from build123d import *

# Parameters (mm, degrees)
SKETCH1_W                   = 33.528
SKETCH1_H                   = 33.02
BOSS_EXTRUDE1_DEPTH         = 3.175
CUT_EXTRUDE1_DEPTH          = 24.742207585
CUT_EXTRUDE2_DEPTH          = 24.742207585
SKETCH4_W                   = 6.08076
SKETCH4_H                   = 5.45338
BOSS_EXTRUDE2_DEPTH         = 6.08076
SKETCH5_W                   = 6.08076
SKETCH5_H                   = 5.45338
BOSS_EXTRUDE3_DEPTH         = 6.08076
SKETCH6_W                   = 6.08076
SKETCH6_H                   = 5.45338
BOSS_EXTRUDE4_DEPTH         = 6.08076
SKETCH7_W                   = 6.08076
SKETCH7_H                   = 5.45338
BOSS_EXTRUDE5_DEPTH         = 6.08076
HOLE1_D                     = 12.7254
M2_5_CLEARANCE_HOLE1_D      = 2.7051
M3_CLEARANCE_HOLE1_D        = 3.556
M2_5_CLEARANCE_HOLE2_D      = 2.7051
M2_5_CLEARANCE_HOLE2_DEPTH  = 39.60876
M2_5_CLEARANCE_HOLE3_D      = 2.7051
M2_5_CLEARANCE_HOLE3_DEPTH  = 39.60876
M2_5_CLEARANCE_HOLE4_REACH  = 27.061
M2_5_CLEARANCE_HOLE4_BORE_R = 1.35255
FILLET1_R                   = 0.635
FILLET2_R                   = 3.04038


with BuildPart() as part:
    # Sketch1 → Boss-Extrude1 (new body)
    with BuildSketch(Plane(origin=(0, 3.175, 0), x_dir=(1, 0, 0), z_dir=(0, 1, 0))):
        Rectangle(SKETCH1_W, SKETCH1_H)
    extrude(amount=-BOSS_EXTRUDE1_DEPTH)

    # Sketch2 → Cut-Extrude1 (cut, through all)
    with BuildSketch(Plane.XZ):
        with BuildLine():
            Line((16.764, -10.42924), (16.764, 10.42924))
            ThreePointArc((16.764, 10.42924), (14.617411383, 9.536940757), (13.7287, 7.388864244))
            Line((13.7287, 7.388864244), (13.7287, -7.388864244))
            ThreePointArc((13.7287, -7.388864244), (14.617411383, -9.536940757), (16.764, -10.42924))
        make_face()
    extrude(amount=-CUT_EXTRUDE1_DEPTH, mode=Mode.SUBTRACT)

    # Sketch3 → Cut-Extrude2 (cut, through all)
    with BuildSketch(Plane.XZ):
        with BuildLine():
            Line((-16.764, 10.42924), (-16.764, -10.42924))
            ThreePointArc((-16.764, -10.42924), (-14.617411383, -9.536940757), (-13.7287, -7.388864244))
            Line((-13.7287, -7.388864244), (-13.7287, 7.388864244))
            ThreePointArc((-13.7287, 7.388864244), (-14.617411383, 9.536940757), (-16.764, 10.42924))
        make_face()
    extrude(amount=-CUT_EXTRUDE2_DEPTH, mode=Mode.SUBTRACT)

    # Sketch4 → Boss-Extrude2 (add)
    with BuildSketch(Plane(origin=(0, 0, -16.51), x_dir=(-1, 0, 0), z_dir=(0, 0, -1))):
        with Locations((13.72362, 5.90169)):
            Rectangle(SKETCH4_W, SKETCH4_H)
    extrude(amount=-BOSS_EXTRUDE2_DEPTH)

    # Sketch5 → Boss-Extrude3 (add)
    with BuildSketch(Plane(origin=(0, 0, -16.51), x_dir=(-1, 0, 0), z_dir=(0, 0, -1))):
        with Locations((-13.72362, 5.90169)):
            Rectangle(SKETCH5_W, SKETCH5_H)
    extrude(amount=-BOSS_EXTRUDE3_DEPTH)

    # Sketch6 → Boss-Extrude4 (add)
    with BuildSketch(Plane.XY.offset(16.51)):
        with Locations((13.72362, 5.90169)):
            Rectangle(SKETCH6_W, SKETCH6_H)
    extrude(amount=-BOSS_EXTRUDE4_DEPTH)

    # Sketch7 → Boss-Extrude5 (add)
    with BuildSketch(Plane.XY.offset(16.51)):
        with Locations((-13.72362, 5.90169)):
            Rectangle(SKETCH7_W, SKETCH7_H)
    extrude(amount=-BOSS_EXTRUDE5_DEPTH)

    # Hole1 (through all)
    with Locations(Plane(origin=(0, 3.175, 0), x_dir=(1, 0, 0), z_dir=(0, 1, 0))):
        with Locations((0, 0)):
            Hole(HOLE1_D / 2)

    # M2.5 Clearance Hole1 (through all)
    with Locations(Plane(origin=(0, 3.175, 0), x_dir=(1, 0, 0), z_dir=(0, 1, 0))):
        with Locations((0, 9.779), (-9.779, 0), (0, -9.779), (9.779, 0)):
            Hole(M2_5_CLEARANCE_HOLE1_D / 2)

    # M3 Clearance Hole1 (through all)
    with Locations(Plane(origin=(0, 3.175, 0), x_dir=(1, 0, 0), z_dir=(0, 1, 0))):
        with Locations((-5.579615818, -13.470384182), (5.579615818, -13.470384182), (5.579615818, 13.470384182), (-5.579615818, 13.470384182), (6.914797213, 6.914797213), (-6.914797213, 6.914797213), (-6.914797213, -6.914797213), (6.914797213, -6.914797213)):
            Hole(M3_CLEARANCE_HOLE1_D / 2)

    # M2.5 Clearance Hole2
    with Locations(Plane(origin=(16.764, 0, 0), x_dir=(0, 0, -1), z_dir=(1, 0, 0))):
        with Locations((-13.470384182, 5.588)):
            Hole(M2_5_CLEARANCE_HOLE2_D / 2, depth=M2_5_CLEARANCE_HOLE2_DEPTH)

    # M2.5 Clearance Hole3
    with Locations(Plane.ZY.offset(16.764)):
        with Locations((-13.470384182, 5.588)):
            Hole(M2_5_CLEARANCE_HOLE3_D / 2, depth=M2_5_CLEARANCE_HOLE3_DEPTH)

    # M2.5 Clearance Hole4 bore → M2.5 Clearance Hole4 (cut, up to next)
    with BuildSketch(Plane(origin=(0, 0, 0), x_dir=(-1, 0, 0), z_dir=(0, -1, 0)), mode=Mode.PRIVATE) as m2_5_clearance_hole4_sk1:
        with Locations((13.470384182, 13.470384182)):
            Circle(M2_5_CLEARANCE_HOLE4_BORE_R)
    m2_5_clearance_hole4_tool1 = extrude(m2_5_clearance_hole4_sk1.sketch, amount=-M2_5_CLEARANCE_HOLE4_REACH, mode=Mode.PRIVATE) & part.part
    # M2.5 Clearance Hole4 bore → M2.5 Clearance Hole4 (cut, up to next)
    with BuildSketch(Plane(origin=(0, 0, 0), x_dir=(-1, 0, 0), z_dir=(0, -1, 0)), mode=Mode.PRIVATE) as m2_5_clearance_hole4_sk2:
        with Locations((-13.470384182, 13.470384182)):
            Circle(M2_5_CLEARANCE_HOLE4_BORE_R)
    m2_5_clearance_hole4_tool2 = extrude(m2_5_clearance_hole4_sk2.sketch, amount=-M2_5_CLEARANCE_HOLE4_REACH, mode=Mode.PRIVATE) & part.part
    # M2.5 Clearance Hole4 bore → M2.5 Clearance Hole4 (cut, up to next)
    with BuildSketch(Plane(origin=(0, 0, 0), x_dir=(-1, 0, 0), z_dir=(0, -1, 0)), mode=Mode.PRIVATE) as m2_5_clearance_hole4_sk3:
        with Locations((-13.470384182, -13.470384182)):
            Circle(M2_5_CLEARANCE_HOLE4_BORE_R)
    m2_5_clearance_hole4_tool3 = extrude(m2_5_clearance_hole4_sk3.sketch, amount=-M2_5_CLEARANCE_HOLE4_REACH, mode=Mode.PRIVATE) & part.part
    # M2.5 Clearance Hole4 bore → M2.5 Clearance Hole4 (cut, up to next)
    with BuildSketch(Plane(origin=(0, 0, 0), x_dir=(-1, 0, 0), z_dir=(0, -1, 0)), mode=Mode.PRIVATE) as m2_5_clearance_hole4_sk4:
        with Locations((13.470384182, -13.470384182)):
            Circle(M2_5_CLEARANCE_HOLE4_BORE_R)
    m2_5_clearance_hole4_tool4 = extrude(m2_5_clearance_hole4_sk4.sketch, amount=-M2_5_CLEARANCE_HOLE4_REACH, mode=Mode.PRIVATE) & part.part
    add(m2_5_clearance_hole4_tool1.solids().sort_by_distance((-13.470384, 0, -13.470384))[0], mode=Mode.SUBTRACT)
    add(m2_5_clearance_hole4_tool2.solids().sort_by_distance((13.470384, 0, -13.470384))[0], mode=Mode.SUBTRACT)
    add(m2_5_clearance_hole4_tool3.solids().sort_by_distance((13.470384, 0, 13.470384))[0], mode=Mode.SUBTRACT)
    add(m2_5_clearance_hole4_tool4.solids().sort_by_distance((-13.470384, 0, 13.470384))[0], mode=Mode.SUBTRACT)

    # Fillet1
    fillet1_edges = [part.edges().sort_by_distance(p)[0] for p in [
        (-16.764, 4.31419, 16.51),
        (-16.764, 4.31419, -16.51),
        (16.764, 4.31419, -16.51),
        (16.764, 4.31419, 16.51),
    ]]
    fillet(fillet1_edges, radius=FILLET1_R)

    # Fillet2
    # the kernel refuses this fillet: 3.04038 mm, written as the material it takes off along each edge
    with BuildSketch(Plane(origin=(-10.68324, 16.22933, -10.42924), x_dir=(-1, 0, 0), z_dir=(0, -1, 0)), Plane(origin=(10.68324, 16.22933, 10.42924), x_dir=(1, 0, 0), z_dir=(0, -1, 0)), Plane(origin=(-10.68324, 3.175, 10.42924), x_dir=(-1, 0, 0), z_dir=(0, 1, 0))) as fillet2_piece_1:
        with BuildLine():
            CenterArc((FILLET2_R, FILLET2_R), FILLET2_R, 180, 90)
            Line((0, FILLET2_R), (0, 0))
            Line((0, 0), (FILLET2_R, 0))
        make_face()
    extrude(amount=13.05433, mode=Mode.SUBTRACT)
    with BuildSketch(Plane(origin=(10.68324, 3.175, -10.42924), x_dir=(0, 0, -1), z_dir=(0, 1, 0))) as fillet2_piece_2:
        with BuildLine():
            CenterArc((FILLET2_R, -FILLET2_R), FILLET2_R, 90, 90)
            Line((0, -FILLET2_R), (0, 0))
            Line((0, 0), (FILLET2_R, 0))
        make_face()
    extrude(amount=13.05433, mode=Mode.SUBTRACT)


solid = part.part
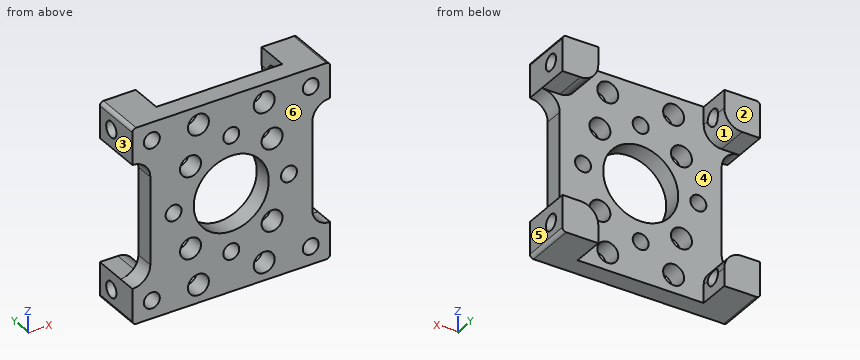
Source: CAD feature listing. Evaluate the final solid. Frame: model axes, mm. Face numbers are marked on the shaded views. A direction names the side the tool comes from. Coordinates: 2 decimals unless noted, no trailing zeros. Write each loop counter-clockwise with the first axis right and the second up, starting at its lowest first coordinate (ties: lowest second). Pieces come first, ordered by that corner, then holes. Notation, with made-up numbers: M 28.5,40.5 L 84.5,40.5 A3 ccw 84.5,45.5 Z; hole C 60.25,52 d7. An arc over 180 degrees is marked long. Use a Markdown table: item, result.
1) Section A-A, the plane z = 0. Output: boundary loops of the cut face in (x, y) (3 decimals).
Conclusion:
| item | result |
|---|---|
| outline | M -13.729,0 L -11.132,0 L -11.132,3.175 L -13.729,3.175 Z; M -8.426,0 L -6.363,0 L -6.363,3.175 L -8.426,3.175 Z; M 6.363,0 L 8.426,0 L 8.426,3.175 L 6.363,3.175 Z; M 11.132,0 L 13.729,0 L 13.729,3.175 L 11.132,3.175 Z |
2) Reachability of the marked faces 1 and 2 from +Z, -Z, +X, -X, +Y, -Y: full face, straight path, thin tool, end or side. Return the list, or none.
Conclusion:
| item | result |
|---|---|
| face 1 | +Y |
| face 2 | +Z, -Z, +X, -X, +Y |
3) Ray query, L1, parallel to Z at x = 13.5, y = 2.25; L2, parallel to X at y = 1, z = 8; L3, parallel to X at y = 2.5, z = 14. Return the intervals inside material, ascending.
Conclusion:
| item | result |
|---|---|
| L1 | z = -16.51 to -14.82, -12.12 to 12.12, 14.82 to 16.51 |
| L2 | x = -13.79 to -8.32, -5.51 to 5.51, 8.32 to 13.79 |
| L3 | x = -16.76 to -14.71, -12.23 to -7.28, -3.88 to 3.88, 7.28 to 12.23, 14.71 to 16.76 |
4) Section D-D, the plane z = -4.5. Output: boundary loops of the cut face in (x, y) (3 decimals), then the cut area to 3 significant figures.
Conclusion:
| item | result |
|---|---|
| outline | M -13.729,0 L -4.498,0 L -4.498,3.175 L -13.729,3.175 Z; M 4.498,0 L 13.729,0 L 13.729,3.175 L 4.498,3.175 Z |
| area | 58.6 mm^2 |
5) First-contact query: pin 1 Ø5 at (x, z) = (-6, 8) entering from +Y (3 decimals); pin 2 Ø2 at (y, z) = (5.59, -13.47) entering from +X; pin 3 Ø1 at (y, z) = (1.5, 6) entering from +X; pin 4 Ø1.6 at (y, z) = (1, 1) entering from -X. Flat tips, straight axial feed; report the tip coordinate or a pass-through.
Conclusion:
| item | result |
|---|---|
| pin 1 | stops at y = 3.175 |
| pin 2 | passes through |
| pin 3 | stops at x = 13.73 |
| pin 4 | stops at x = -13.73 |
6) Section B-B, the plane x = 0. Output: boundary loops of the cut face in (y, z) (3 decimals), then the cut area to 3 significant figures.
Conclusion:
| item | result |
|---|---|
| outline | M 0,-16.51 L 3.175,-16.51 L 3.175,-11.132 L 0,-11.132 Z; M 0,-8.426 L 3.175,-8.426 L 3.175,-6.363 L 0,-6.363 Z; M 0,6.363 L 3.175,6.363 L 3.175,8.426 L 0,8.426 Z; M 0,11.132 L 3.175,11.132 L 3.175,16.51 L 0,16.51 Z |
| area | 47.3 mm^2 |
7) Section C-C, the plane y = 8. Output: boundary loops of the cut face in (x, z) (3 decimals), then the cut area to 3 significant figures.
Conclusion:
| item | result |
|---|---|
| outline | M -16.764,-15.875 A0.635 ccw -16.129,-16.51 L -10.683,-16.51 L -10.683,-13.47 A3.04 ccw -13.724,-10.429 L -16.764,-10.429 Z; M -16.764,10.429 L -13.724,10.429 A3.04 ccw -10.683,13.47 L -10.683,16.51 L -16.129,16.51 A0.635 ccw -16.764,15.875 Z; M 10.683,-16.51 L 16.129,-16.51 A0.635 ccw 16.764,-15.875 L 16.764,-10.429 L 13.724,-10.429 A3.04 ccw 10.683,-13.47 Z; M 10.683,13.47 A3.04 ccw 13.724,10.429 L 16.764,10.429 L 16.764,15.875 A0.635 ccw 16.129,16.51 L 10.683,16.51 Z |
| area | 140 mm^2 |
8) Mould query, pull axis X, two halves, no side actions, for the marked faces 3, 4, 5 and 6. Classes: pulls with the +X half, pulls with the -X half, needs draft (parallel to the pull), parting line crosses it, or undercut.
Conclusion:
| item | result |
|---|---|
| face 3 | pulls with the -X half |
| face 4 | undercut |
| face 5 | pulls with the +X half |
| face 6 | needs draft |
